```python
from build123d import *

# Parameters (mm, degrees)
PAD_DEPTH    = 10
PAD001_DEPTH = 9
PAD002_DEPTH = 9
PAD003_DEPTH = 8
PAD004_DEPTH = 8
PAD005_DEPTH = 12.5
PAD006_DEPTH = 12.5


with BuildPart() as part:
    # Sketch → Pad (new body)
    with BuildSketch(Plane.XY):
        with BuildLine():
            ThreePointArc((0, -5), (5, 0), (0, 5))
            ThreePointArc((0, 5), (-5, 0), (0, -5))
        make_face()
    extrude(amount=-PAD_DEPTH)

    # Pad Face3 → Pad001 (add)
    with BuildSketch(Plane(origin=(0, 0, 0), x_dir=(0, 1, 0), z_dir=(0, 0, 1))):
        with BuildLine():
            ThreePointArc((-5, 0), (0, -5), (5, 0))
            ThreePointArc((5, 0), (0, 5), (-5, 0))
        make_face()
    extrude(amount=PAD001_DEPTH)

    # Pad001 Face4 → Pad002 (add)
    with BuildSketch(Plane(origin=(0, 0, -10), x_dir=(0, -1, 0), z_dir=(0, 0, -1))):
        with BuildLine():
            ThreePointArc((-5, 0), (0, -5), (5, 0))
            ThreePointArc((5, 0), (0, 5), (-5, 0))
        make_face()
    extrude(amount=PAD002_DEPTH)

    # Pad002 Face7 → Pad003 (add)
    with BuildSketch(Plane(origin=(0, 0, 9), x_dir=(0, 1, 0), z_dir=(0, 0, 1))):
        with BuildLine():
            ThreePointArc((-5, 0), (0, -5), (5, 0))
            ThreePointArc((5, 0), (0, 5), (-5, 0))
        make_face()
    extrude(amount=PAD003_DEPTH)

    # Pad003 Face8 → Pad004 (add)
    with BuildSketch(Plane(origin=(0, 0, -19), x_dir=(0, -1, 0), z_dir=(0, 0, -1))):
        with BuildLine():
            ThreePointArc((-5, 0), (0, -5), (5, 0))
            ThreePointArc((5, 0), (0, 5), (-5, 0))
        make_face()
    extrude(amount=PAD004_DEPTH)

    # Pad004 Face11 → Pad005 (add)
    with BuildSketch(Plane(origin=(0, 0, 17), x_dir=(0, 1, 0), z_dir=(0, 0, 1))):
        with BuildLine():
            ThreePointArc((-5, 0), (0, -5), (5, 0))
            ThreePointArc((5, 0), (0, 5), (-5, 0))
        make_face()
    extrude(amount=PAD005_DEPTH)

    # Pad005 Face12 → Pad006 (add)
    with BuildSketch(Plane(origin=(0, 0, -27), x_dir=(0, -1, 0), z_dir=(0, 0, -1))):
        with BuildLine():
            ThreePointArc((-5, 0), (0, -5), (5, 0))
            ThreePointArc((5, 0), (0, 5), (-5, 0))
        make_face()
    extrude(amount=PAD006_DEPTH)


solid = part.part
```
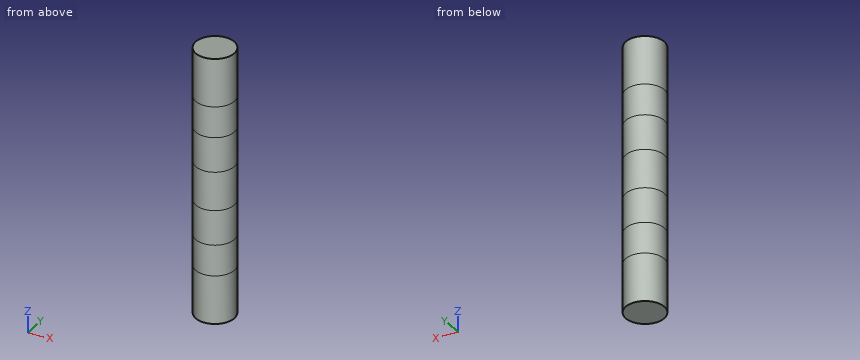
For this review, take the finished solid that the model builds, in its own axes (mm). Round coordinates to 2 decimals unless told otherwise and drop trailing zeros. Write each loop counter-clockwise with the first axis right and the second up, starting at its lowest first coordinate (ties: lowest second). Pieces come first, ordered by that corner, then holes. Notation, with made-up numbers: (-27, 5.5) -> (0, 5.5) arc R19 ccw to (0, 32.5) -> close; hole circle Ø4 at (67, 19). An arc over 180 degrees is marked (long way). Use one line per item in the form item = value.
Q1. Clearance check with flat-ended pins moving along their axes: pin 1 Ø3 at (y, z) = (2, -1.5) entering from +X; pin 2 Ø2 at (x, z) = (-1.5, -17) entering from -Y; pin 3 Ø1 at (y, z) = (-3, -12) entering from +X. State where each tip first meets the part, or that it passes through.
Resolved:
pin_1 = 4.97
pin_2 = -4.97
pin_3 = 4.33
Q2. Consider section B-B (x = -1.25). State the section outline as (y, z) points, then the cut area to 3 significant figures.
Resolved:
outline = (-4.84, -39.5) -> (4.84, -39.5) -> (4.84, 29.5) -> (-4.84, 29.5) -> close
area = 668 mm²
Q3. To check wall thickness, follow probe 1 along X at (y, z) = (-0.25, 1); probe 2 along X at (y, z) = (-2.25, 17). State the ranges of each line that lie inside material, in increasing order. Write a range as from..to.
Resolved:
probe_1 = -4.99..4.99
probe_2 = -4.47..4.47
Q4. Consider section A-A (z = -22). State the section outline as (x, y) points.
Resolved:
outline = circle Ø10 at (0, 0)
